Study the drawing (mm; zero at the part's minimum x, y, z) and answer. A direction names the side the tool comes from. Give positions to 0.01 mm unless a question says otherwise; leave off trailing zeros. Write each loop counter-clockwise with the first axis right and the second up, starting at its lowest first coordinate (ties: lowest second). Pieces come first, ordered by that corner, then holes. Notation, with made-up numbers: (19, 31) -> (29, 31) arc R21 cw to (29, 40) -> close; hole circle Ø3 at (1.5, 11). An arc over 180 degrees is marked (long way). One line per question, with ' | ' between items.
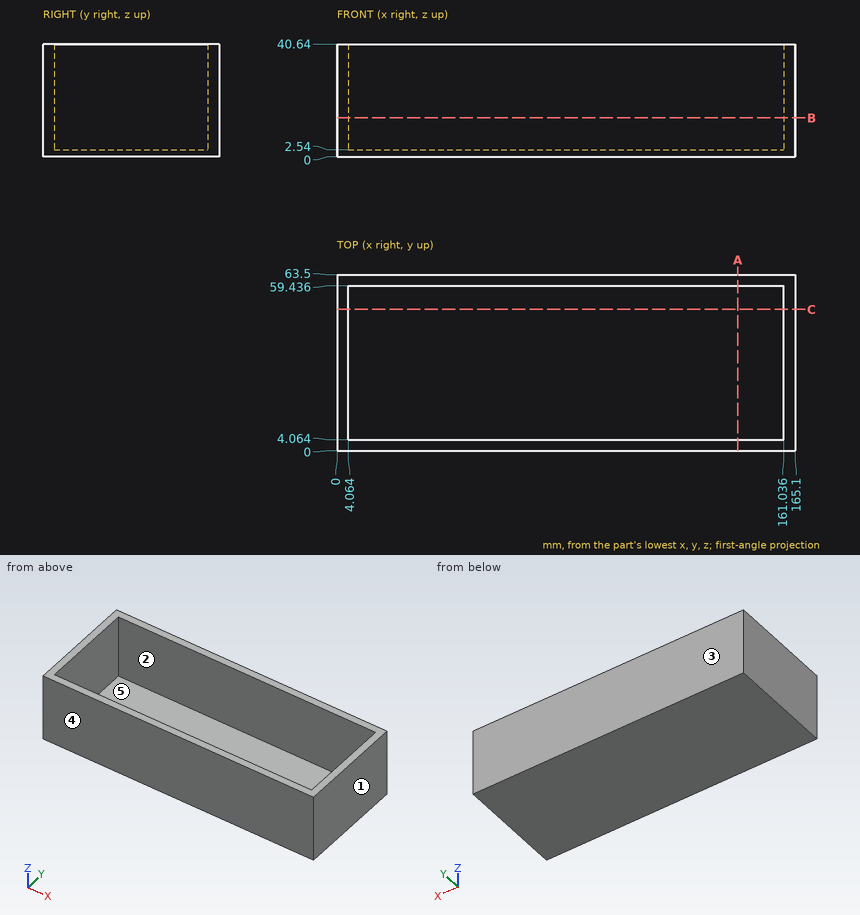
Item 1: Determine the mould class of the marked faces 1, 2 and 3 for opening direction Y: pulls with the +Y half, pulls with the -Y half, needs draft (parallel to the pull), parting line crosses it, or undercut.
Answers below:
face 1: needs draft | face 2: undercut | face 3: pulls with the +Y half
Item 2: A flat-ended cylindrical pin translates along its axis: pin 1 (3 mm diameter, centred on x = 46.5, y = 50.5, fed in from +Z). Find the tip coordinate at first contact, or state that the pin passes through.
Answers below:
pin 1: z = 2.54
Item 3: Find section A-A (x = 144.5). Write down the section's boundary in (y, z).
Answers below:
outline: (0, 0) -> (63.5, 0) -> (63.5, 40.64) -> (59.44, 40.64) -> (59.44, 2.54) -> (4.06, 2.54) -> (4.06, 40.64) -> (0, 40.64) -> close
Item 4: Find section B-B (z = 14). Write down the section's boundary in (x, y).
Answers below:
outline: (0, 0) -> (165.1, 0) -> (165.1, 63.5) -> (0, 63.5) -> close; hole (4.06, 4.06) -> (161.04, 4.06) -> (161.04, 59.44) -> (4.06, 59.44) -> close
Item 5: Find section C-C (y = 51). Write down the section's boundary in (x, z), then the cut area to 3 significant figures.
Answers below:
outline: (0, 0) -> (165.1, 0) -> (165.1, 40.64) -> (161.04, 40.64) -> (161.04, 2.54) -> (4.06, 2.54) -> (4.06, 40.64) -> (0, 40.64) -> close | area: 729 mm²
Item 6: Consider line 1 (Y direction, x = 12, z = 28); line 2 (X direction, y = 47.5, z = 12); line 3 (Z direction, x = 140, y = 22). Determine where each line is inside the solid, lowest interval first. Write a range as [from, to].
Answers below:
line 1: [0, 4.06], [59.44, 63.5] | line 2: [0, 4.06], [161.04, 165.1] | line 3: [0, 2.54]
Item 7: A tool of negligible diameter and unlimited length cuts with its end or side. For the marked faces 4 and 5, from which of +Z, -Z, +X, -X, +Y, -Y can it reach the whole face along a straight path? Write none if from no direction.
Answers below:
face 4: +Z, -Z, +X, -X, -Y | face 5: +Z
